Geometry check sheet. Reference: drawing and pictorial views, mm from the part's lowest x, y, z. Coordinates: 2 decimals unless noted, no trailing zeros. Loops run counter-clockwise (first coordinate to the right, second up) from the corner with the lowest first, then second, coordinate; pieces in that order, holes last. Notation, with made-up numbers: (-15, -17.5) -> (2, -17.5) arc R12 cw to (2, 1.5) -> close; hole circle Ø1 at (56, 87.5). An arc over 180 degrees is marked (long way). Answer as a JSON object with one key per item and string values. Group by question number.
Q1. Cross-section at A-A on y = 13.5. Record the boundary of the cut face in (x, z) (1 decimal).
Q2. Cross-section at B-B on x = 24.5. Record the boundary of the cut face in (y, z) (1 decimal).
Q3. Cross-section at D-D on y = 36. Record the boundary of the cut face in (x, z) (1 decimal).
Q4. Gauge pin test, flat ends, axial feed: pin 1 Ø2 at (y, z) = (9, 4.5) entering from +X; pin 2 Ø1.5 at (y, z) = (18, 4) entering from -X (1 decimal); pin 3 Ø1 at (x, z) = (43, 13) entering from +Y (1 decimal). Record the tip position at first contact, or that the pin passes through.
Q5. Scan lines: L1, parallel to Y at x = 24.5, z = 9 (1 decimal); L2, parallel to X at y = 26, z = 16.75; L3, parallel to X at y = 29.5, z = 9.5. Record each from-to range of solid material in increasing order.
Q6. Release check for a two-part mould opening along X. For the marked faces 1, 2, 3 and 4 record: released by +X, released by -X, zero draft, split by the parting line, or undercut.
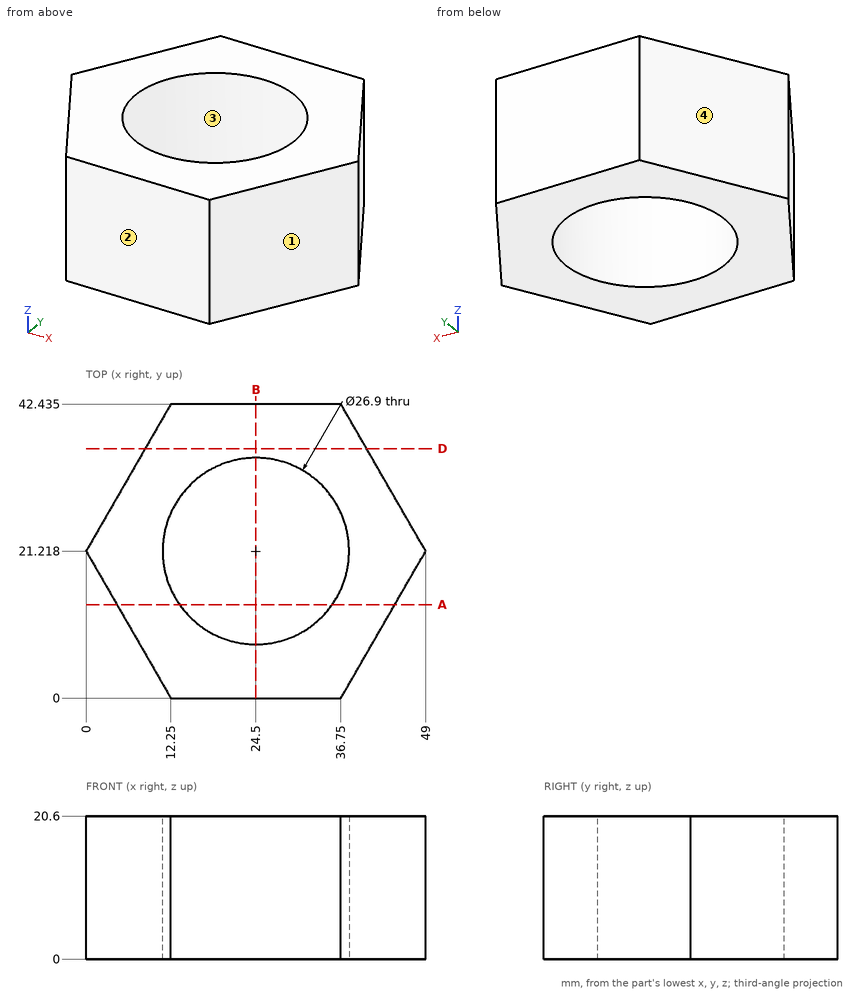
Computed values:
{
 "1": {"outline": "(4.5, 0) -> (13.5, 0) -> (13.5, 20.6) -> (4.5, 20.6) -> close; (35.5, 0) -> (44.5, 0) -> (44.5, 20.6) -> (35.5, 20.6) -> close"},
 "2": {"outline": "(0, 0) -> (7.8, 0) -> (7.8, 20.6) -> (0, 20.6) -> close; (34.7, 0) -> (42.4, 0) -> (42.4, 20.6) -> (34.7, 20.6) -> close"},
 "3": {"outline": "(8.5, 0) -> (40.5, 0) -> (40.5, 20.6) -> (8.5, 20.6) -> close"},
 "4": {"pin 1": "stops at x = 42.52", "pin 2": "stops at x = 1.4", "pin 3": "stops at y = 32.5"},
 "5": {"L1": "y = 0 to 7.8, 34.7 to 42.4", "L2": "x = 2.76 to 11.93, 37.07 to 46.24", "L3": "x = 4.78 to 13.9, 35.1 to 44.22"},
 "6": {"face 1": "released by +X", "face 2": "zero draft", "face 3": "undercut", "face 4": "released by -X"}
}
